Could you check a few things on this model? Use its own coordinates, in mm. A direction names the side the tool comes from. Round coordinates to 2 decimals unless told otherwise and drop trailing zeros. Loops run counter-clockwise (first coordinate to the right, second up) from the corner with the lowest first, then second, coordinate; pieces in that order, holes last. Notation, with made-up numbers: (71, 32.25) - (76, 32.25) arc R14 ccw to (76, 42.25) - close; hole circle Ø7 at (29, -25). An arc over 180 degrees is marked (long way). Use one line per item in the form item = value.
```python
from build123d import *

# Parameters (mm, degrees)
SKETCH1_R                = 0.5
BOSS_EXTRUDE1_DEPTH      = 2.5
FILLET1_R                = 2
FILLET2_R                = 1.5
M2_5X0_45_TAPPED_HOLE1_D = 2.05


with BuildPart() as part:
    # Sketch1 → Boss-Extrude1 (new body)
    with BuildSketch(Plane(origin=(0, 0, 0), x_dir=(1, 0, 0), z_dir=(0, 1, 0))):
        with BuildLine():
            Line((0, 0), (45.5, 0))
            Line((45.5, 0), (45.5, 13.5))
            ThreePointArc((45.5, 13.5), (49, 17), (45.5, 20.5))
            Line((45.5, 20.5), (45.5, 37))
            Line((45.5, 37), (18, 37))
            Line((18, 37), (18, 35.5))
            Line((18, 35.5), (0, 35.5))
            Line((0, 35.5), (0, 0))
        make_face()
        with Locations(Location((45.5, 17, 0), (0, 0, 270))):
            Circle(SKETCH1_R, mode=Mode.SUBTRACT)
        with Locations(Location((6.5, 3, 0), (0, 0, 270))):
            Circle(SKETCH1_R, mode=Mode.SUBTRACT)
        with Locations(Location((6.5, 32.5, 0), (0, 0, 270))):
            Circle(SKETCH1_R, mode=Mode.SUBTRACT)
    extrude(amount=BOSS_EXTRUDE1_DEPTH)

    # Fillet1
    fillet1_edges = [part.edges().sort_by_distance(p)[0] for p in [
        (0, 1.25, -35.5),
        (45.5, 1.25, -37),
        (45.5, 1.25, 0),
        (0, 1.25, 0),
    ]]
    fillet(fillet1_edges, radius=FILLET1_R)

    # Fillet2
    fillet2_edges = [part.edges().sort_by_distance(p)[0] for p in [
        (18, 1.25, -37),
    ]]
    fillet(fillet2_edges, radius=FILLET2_R - 0.0001)  # a hair under: the kernel refuses the full size

    # M2.5x0.45 Tapped Hole1 (through all)
    with Locations(Plane(origin=(0, 2.5, 0), x_dir=(1, 0, 0), z_dir=(0, 1, 0))):
        with Locations((6.5, 32.5), (6.5, 3), (45.5, 17)):
            Hole(M2_5X0_45_TAPPED_HOLE1_D / 2)


solid = part.part
```
1. If we section it at C-C, the plane y = 1.35: Count the separate pieces of the cut face and the enclosed holes in it, plus the area to 3 significant figures.
Solution:
separate_pieces = 1
enclosed_holes = 3
area = 1,660 mm^2
2. For P1, Ø0.8, axis at y = 1, z = -25, coming from the +X side, with a flat end and sliding along its axis, tell me the tip position at first contact or that it passes through.
Solution:
P1 = 45.5
3. If we section it at D-D, the plane z = -32.5: Write out the boundary of the cut face in (x, y) (3 decimals), plus the area to 3 significant figures.
Solution:
outline = (0, 0) - (5.475, 0) - (5.475, 2.5) - (0, 2.5) - close; (7.525, 0) - (45.5, 0) - (45.5, 2.5) - (7.525, 2.5) - close
area = 109 mm^2
4. If we section it at B-B, the plane x = 6.5: Write out the boundary of the cut face in (y, z) (3 decimals).
Solution:
outline = (0, -35.5) - (2.5, -35.5) - (2.5, -33.525) - (0, -33.525) - close; (0, -31.475) - (2.5, -31.475) - (2.5, -4.025) - (0, -4.025) - close; (0, -1.975) - (2.5, -1.975) - (2.5, 0) - (0, 0) - close
5. If we section it at A-A, the plane z = -17: Write out the boundary of the cut face in (x, y) (3 decimals), plus the area to 3 significant figures.
Solution:
outline = (0, 0) - (44.475, 0) - (44.475, 2.5) - (0, 2.5) - close; (46.525, 0) - (49, 0) - (49, 2.5) - (46.525, 2.5) - close
area = 117 mm^2
6. We'd pull the mould along X, two halves only. Please class faces 4 (the face through (22, 1, 0)), 5 (the face through (0, 1, -18)), 6 (the face through (45.5, 1, -28)), 7 (the face through (7.524, 1.233, -3.045)): +X half, -X half, draft (parallel to the pull), parting line (faces both ways), or undercut.
Solution:
face_4 = draft
face_5 = -X half
face_6 = +X half
face_7 = undercut
7. On a 3-axis mill with a long thin cutter (end or side, diameter ignored), from which of +Z, -Z, +X, -X, +Y, -Y can I reach the whole of each face in a straight line? I mean faces 1 (the face through (45.5, 1, -8)), 2 (the face through (24, 0, -19)), 3 (the face through (10, 1, -35.5)). Say none if no direction works.
Solution:
face_1 = +Z, +X, +Y, -Y
face_2 = +Z, -Z, +X, -X, -Y
face_3 = -Z, -X, +Y, -Y
8. Please list where these lines run through material, in increasing order: line 1 along Z through (x, y) = (6.5, 1.45) (3 decimals); line 2 along X through (y, z) = (1, -17) (3 decimals); line 3 along X through (y, z) = (0.6, -32.5) (3 decimals).
Solution:
line_1 = -35.5 to -33.525, -31.475 to -4.025, -1.975 to 0
line_2 = 0 to 44.475, 46.525 to 49
line_3 = 0 to 5.475, 7.525 to 45.5
